```python
from build123d import *

# Parameters (mm, degrees)
BOSS_EXTRUDE2_DEPTH = 35
SKETCH3_R           = 11
SKETCH3_R_2         = 1.75
BOSS_EXTRUDE5_DEPTH = 3.15
CUT_EXTRUDE2_REACH  = 122.042
SKETCH5_R           = 1.75
SKETCH6_R           = 2.5
CUT_EXTRUDE3_DEPTH  = 2.15
CUT_EXTRUDE4_REACH  = 124.883
SKETCH7_R           = 4
CHAMFER1_SIZE       = 4


with BuildPart() as part:
    # Sketch1 → Boss-Extrude2 (new body)
    with BuildSketch(Plane(origin=(0, 0, 0), x_dir=(1, 0, 0), z_dir=(0, 1, 0))):
        Polygon((0, 0), (0, 39), (108, 39), (108, 0), (103, 0), (103, 34), (5, 34), (5, 0), align=None)
    extrude(amount=BOSS_EXTRUDE2_DEPTH)

    # Sketch3 → Boss-Extrude5 (add)
    with BuildSketch(Plane(origin=(108, 0, 0), x_dir=(0, 0, -1), z_dir=(1, 0, 0))):
        with Locations(Location((16, 17.5, 0), (0, 0, 180))):
            Circle(SKETCH3_R)
        with Locations((16, 9.5)):
            Circle(SKETCH3_R_2, mode=Mode.SUBTRACT)
        with Locations((8, 17.5)):
            Circle(SKETCH3_R_2, mode=Mode.SUBTRACT)
        with Locations((16, 25.5)):
            Circle(SKETCH3_R_2, mode=Mode.SUBTRACT)
        with Locations((24, 17.5)):
            Circle(SKETCH3_R_2, mode=Mode.SUBTRACT)
    extrude(amount=BOSS_EXTRUDE5_DEPTH)

    # Sketch5 → Cut-Extrude2 (cut, up to next)
    with BuildSketch(Plane(origin=(108, 0, 0), x_dir=(0, 0, -1), z_dir=(1, 0, 0)), mode=Mode.PRIVATE) as cut_extrude2_sk1:
        with Locations((16, 9.5)):
            Circle(SKETCH5_R)
    cut_extrude2_tool1 = extrude(cut_extrude2_sk1.sketch, amount=-CUT_EXTRUDE2_REACH, mode=Mode.PRIVATE) & part.part
    # Sketch5 → Cut-Extrude2 (cut, up to next)
    with BuildSketch(Plane(origin=(108, 0, 0), x_dir=(0, 0, -1), z_dir=(1, 0, 0)), mode=Mode.PRIVATE) as cut_extrude2_sk2:
        with Locations((24, 17.5)):
            Circle(SKETCH5_R)
    cut_extrude2_tool2 = extrude(cut_extrude2_sk2.sketch, amount=-CUT_EXTRUDE2_REACH, mode=Mode.PRIVATE) & part.part
    # Sketch5 → Cut-Extrude2 (cut, up to next)
    with BuildSketch(Plane(origin=(108, 0, 0), x_dir=(0, 0, -1), z_dir=(1, 0, 0)), mode=Mode.PRIVATE) as cut_extrude2_sk3:
        with Locations((16, 25.5)):
            Circle(SKETCH5_R)
    cut_extrude2_tool3 = extrude(cut_extrude2_sk3.sketch, amount=-CUT_EXTRUDE2_REACH, mode=Mode.PRIVATE) & part.part
    # Sketch5 → Cut-Extrude2 (cut, up to next)
    with BuildSketch(Plane(origin=(108, 0, 0), x_dir=(0, 0, -1), z_dir=(1, 0, 0)), mode=Mode.PRIVATE) as cut_extrude2_sk4:
        with Locations((8, 17.5)):
            Circle(SKETCH5_R)
    cut_extrude2_tool4 = extrude(cut_extrude2_sk4.sketch, amount=-CUT_EXTRUDE2_REACH, mode=Mode.PRIVATE) & part.part
    add(cut_extrude2_tool1.solids().sort_by_distance((108, 9.5, -16))[0], mode=Mode.SUBTRACT)
    add(cut_extrude2_tool2.solids().sort_by_distance((108, 17.5, -24))[0], mode=Mode.SUBTRACT)
    add(cut_extrude2_tool3.solids().sort_by_distance((108, 25.5, -16))[0], mode=Mode.SUBTRACT)
    add(cut_extrude2_tool4.solids().sort_by_distance((108, 17.5, -8))[0], mode=Mode.SUBTRACT)

    # Sketch6 → Cut-Extrude3 (cut)
    with BuildSketch(Plane.ZY.offset(-103)):
        with Locations((-16, 9.5)):
            Circle(SKETCH6_R)
        with Locations((-24, 17.5)):
            Circle(SKETCH6_R)
        with Locations((-16, 25.5)):
            Circle(SKETCH6_R)
        with Locations((-8, 17.5)):
            Circle(SKETCH6_R)
    extrude(amount=-CUT_EXTRUDE3_DEPTH, mode=Mode.SUBTRACT)

    # Sketch7 → Cut-Extrude4 (cut, up to next)
    with BuildSketch(Plane.ZY, mode=Mode.PRIVATE) as cut_extrude4_sk1:
        with Locations((-16, 17.5)):
            Circle(SKETCH7_R)
    cut_extrude4_tool1 = extrude(cut_extrude4_sk1.sketch, amount=-CUT_EXTRUDE4_REACH, mode=Mode.PRIVATE) & part.part
    add(cut_extrude4_tool1.solids().sort_by_distance((0, 17.5, -16))[0], mode=Mode.SUBTRACT)

    # Chamfer1
    chamfer1_edges = [part.edges().sort_by_distance(p)[0] for p in [
        (103, 17.5, -34),
        (5, 17.5, -34),
    ]]
    chamfer(chamfer1_edges, length=CHAMFER1_SIZE)


solid = part.part
```
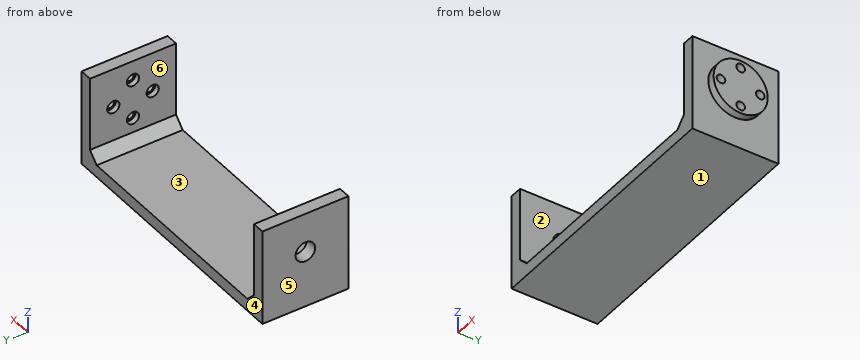
Build history of the part. All positions in model axes, mm. Face numbers are marked on the shaded views. A direction names the side the tool comes from. Round coordinates to 2 decimals unless told otherwise and drop trailing zeros. Loops run counter-clockwise (first coordinate to the right, second up) from the corner with the lowest first, then second, coordinate; pieces in that order, holes last.
Item 1: Saw through at A-A (z = -31). List the corners of the cut face in (x, y).
Item 2: Drill centre lines: line 1 along Y through (x, z) = (105.9, -16); line 2 along Y through (x, z) = (103.85, -16); line 3 along X through (y, z) = (29, -22). Where is each one in solid material? Low to high.
Item 3: Saw through at B-B (y = 17.5). State how many separate pieces and enclosed holes the cut face has, then the cut area to 3 significant figures.
Item 4: Which spindle directions (+Z, -Z, +X, -X, +Y, -Y) get a long thin tool onto all of the face, cutting with end or side? Do the marked faces 1 and 2. Say none if no direction does.
Item 5: Pin check, flat tips, straight feed: P1, Ø1.5, axis at y = 8, z = -30, coming from the -X side; P2, Ø2, axis at y = 17.5, z = -24, coming from the +X side; P3, Ø1.5, axis at x = 41, y = 9, coming from the +Z side. Stop position of each tip, or through.
Item 6: Saw through at C-C (y = 30). List the corners of the cut face in (x, z), then the cut area to 3 significant figures.
Item 7: Saw through at D-D (z = -24.5). List the corners of the cut face in (x, y).
Item 8: Two-plate mould, pull along X, no slides. Class the marked faces 3, 4, 5 and 6: released by +X, released by -X, zero draft, split by the parting line, or undercut.
Worked answers:
1. outline: (0, 0) - (6, 0) - (6, 35) - (0, 35) - close; (102, 0) - (108, 0) - (108, 35) - (102, 35) - close
2. line 1: y = 0 to 7.75, 11.25 to 23.75, 27.25 to 35
2. line 2: y = 0 to 7, 12 to 23, 28 to 35
2. line 3: x = 0 to 5, 103 to 108
3. separate pieces: 4
3. enclosed holes: 0
3. area: 862 mm2
4. face 1: -Z, +X, -X, +Y, -Y
4. face 2: +Z, +Y, -Y
5. P1: stops at x = 0
5. P2: stops at x = 5
5. P3: stops at z = -34
6. outline: (0, -39) - (108, -39) - (108, 0) - (103, 0) - (103, -30) - (99, -34) - (9, -34) - (5, -30) - (5, 0) - (0, 0) - close
6. area: 896 mm2
7. outline: (0, 0) - (5, 0) - (5, 35) - (0, 35) - close; (103, 0) - (108, 0) - (108, 10.52) - (111.15, 10.52) - (111.15, 15.82) - (105.15, 15.82) - (105.15, 15.05) - (103, 15.05) - close; (103, 19.95) - (105.15, 19.95) - (105.15, 19.18) - (111.15, 19.18) - (111.15, 24.48) - (108, 24.48) - (108, 35) - (103, 35) - close
8. face 3: undercut
8. face 4: zero draft
8. face 5: released by -X
8. face 6: undercut
